Part model, mm, in its own coordinate system. Face numbers are marked on the shaded views. A direction names the side the tool comes from. Round coordinates to 2 decimals unless told otherwise and drop trailing zeros. Write each loop counter-clockwise with the first axis right and the second up, starting at its lowest first coordinate (ties: lowest second). Pieces come first, ordered by that corner, then holes. Notation, with made-up numbers: M 44,56 L 91,56 A25 cw 91,95 Z; hole C -19.75,67.5 d11. An arc over 180 degrees is marked long. Answer as a JSON object with one key per item and string values. Group by question number.
1. Which spindle directions (+Z, -Z, +X, -X, +Y, -Y) get a long thin tool onto all of the face, cutting with end or side? Do the marked faces 4 and 5. Say none if no direction does.
2. Drill centre lines: line 1 (Y direction, x = 13, z = 6); line 2 (Y direction, x = 15, z = 25); line 3 (Z direction, x = 51, y = -10). Where is each one in solid material? Low to high. Write a range as from..to.
3. Band-saw the part on D-D, the plane y = -7.5. Write the cut outline in (x, z).
4. Drop flat-ended pins along their axis: pin 1 (12 mm diameter, centred on x = 49, z = 25, fed in from -Y); pin 2 (1 mm diameter, centred on x = 60, y = -12.5, fed in from +Z); pin 3 (10 mm diameter, centred on x = 33, z = 3, fed in from -Y); pin 4 (6.5 mm diameter, centred on x = 13, y = -24, fed in from -Z). Give the stop position or say it passes through.
5. Two-plate mould, pull along Y, no slides. Class the marked faces 1, 2 and 3: +Y half, -Y half, draft (parallel to the pull), parting line (faces both ways), or undercut.
6. Band-saw the part on B-B, the plane y = -34. Write the cut outline in (x, z), plus the area to 3 significant figures.
7. Band-saw the part on A-A, the plane y = -12. Write the cut outline in (x, z), plus the area to 3 significant figures.
8. Band-saw the part on C-C, the plane x = 25. Write the cut outline in (y, z), plus the area to 3 significant figures.
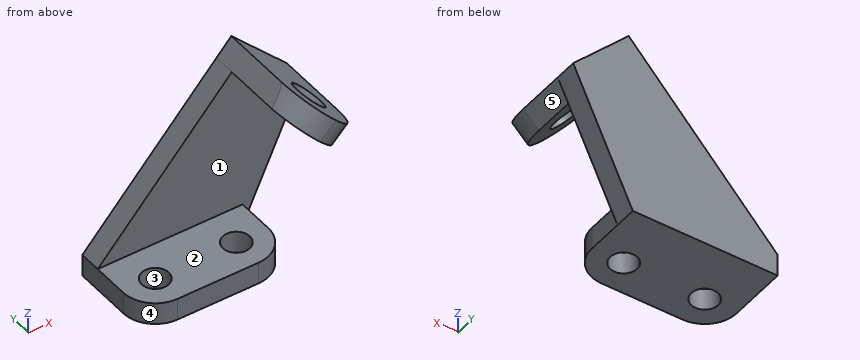
from build123d import *

# Parameters (mm, degrees)
F0_W       = 59
F0_H       = 9
F1_DEPTH   = 37
F2_R       = 5.5
F3_DEPTH   = 25
F5_DEPTH   = 9
F6_DEPTH   = 45
F7_R       = 7
F6_FACE1_W = 36
F6_FACE1_H = 9
F8_DEPTH   = 25
F9_R       = 13


with BuildPart() as f1:
    # F0 (on Front) → F1 (new body)
    with BuildSketch(Plane.XZ):
        with Locations((29.5, 4.5)):
            Rectangle(F0_W, F0_H)
    extrude(amount=F1_DEPTH)

    # F2 (on face) → F3 (cut)
    with BuildSketch(Plane.XY.offset(9)):
        with Locations((46, -24)):
            Circle(F2_R)
        with Locations((13, -24)):
            Circle(F2_R)
    extrude(amount=-F3_DEPTH, mode=Mode.SUBTRACT)

    # F4 (on face) → F5 (join)
    with BuildSketch(Plane(origin=(0, 0, 0), x_dir=(-1, 0, 0), z_dir=(0, 1, 0))):
        Polygon((-77.2376988573, 46.0468557694), (-83.313708499, 52.686291501), (-59, 0), (-59, 9), (0, 9), (-54.6102818594, 68.6742727673), align=None)
    extrude(amount=-F5_DEPTH)

    # F4 (on face) → F6 (join)
    with BuildSketch(Plane(origin=(0, 0, 0), x_dir=(-1, 0, 0), z_dir=(0, 1, 0))):
        Polygon((-60.686291501, 75.313708499), (-72, 64), (-83.313708499, 52.686291501), (-77.2376988573, 46.0468557694), (-54.6102818594, 68.6742727673), align=None)
    extrude(amount=-F6_DEPTH)

    # F7 (on face) + F6_face1 (on face) → F8 (cut)
    with BuildSketch(Plane(origin=(68, 0, 68), x_dir=(0, 1, 0), z_dir=(0.7071067812, 0, 0.7071067812))):
        with Locations((-29, -5.6568542495)):
            Circle(F7_R)
        with BuildLine():
            ThreePointArc((-45, -5.6568542495), (-40.313708499, 5.6568542495), (-29, 10.3431457505))
            Line((-29, 10.3431457505), (-45, 10.3431457505))
            Line((-45, 10.3431457505), (-45, -5.6568542495))
        make_face()
        with BuildLine():
            ThreePointArc((-29, -21.6568542495), (-40.313708499, -16.9705627485), (-45, -5.6568542495))
            Line((-45, -5.6568542495), (-45, -21.6568542495))
            Line((-45, -21.6568542495), (-29, -21.6568542495))
        make_face()
    with BuildSketch(Plane(origin=(80.2757036782, -27, 49.3665736352), x_dir=(0, 1, 0), z_dir=(0.7377150813, 0, -0.6751121824))):
        Rectangle(F6_FACE1_W, F6_FACE1_H)
    extrude(amount=-F8_DEPTH, dir=(0.7071067812, 0, 0.7071067812), mode=Mode.SUBTRACT)

    # F9
    f9_edges = [f1.edges().sort_by_distance(p)[0] for p in [
        (59, -37, 4.5),
        (0, -37, 4.5),
    ]]
    fillet(f9_edges, radius=F9_R)


solid = f1.part
Worked answers:
{
 "1": {"face 4": "+Z, -Z, -X, -Y", "face 5": "-Z, +X, -Y"},
 "2": {"line 1": "y = -37..-29.5, -18.5..0", "line 2": "y = -9..0", "line 3": "z = 0..9"},
 "3": {"outline": "M 0,0 L 59,0 L 83.31,52.69 L 60.69,75.31 L 0,9 Z"},
 "4": {"pin 1": "stops at y = -9", "pin 2": "stops at z = 75.11", "pin 3": "stops at y = -37", "pin 4": "passes through"},
 "5": {"face 1": "-Y half", "face 2": "draft", "face 3": "undercut"},
 "6": {"outline": "M 4.69,0 L 54.31,0 L 54.31,9 L 4.69,9 Z; M 54.9,68.39 L 62.18,61.11 L 68.54,67.46 L 61.25,74.75 Z; M 69.11,54.18 L 76.39,46.9 L 82.75,53.25 L 75.46,60.54 Z", "area": "632 mm^2"},
 "7": {"outline": "M 0,0 L 59,0 L 59,9 L 0,9 Z; M 54.61,68.67 L 76.96,46.33 L 83.31,52.69 L 60.69,75.31 Z", "area": "817 mm^2"},
 "8": {"outline": "M -37,0 L 0,0 L 0,36.32 L -9,36.32 L -9,9 L -37,9 Z", "area": "579 mm^2"}
}
